Could you check a few things on this model? Use its own coordinates, in mm. A direction names the side the tool comes from. Round coordinates to 2 decimals unless told otherwise and drop trailing zeros. Loops run counter-clockwise (first coordinate to the right, second up) from the corner with the lowest first, then second, coordinate; pieces in that order, holes last. Notation, with made-up numbers: (-19.5, 71.5) -> (10.5, 71.5) arc R21 cw to (10.5, 96.5) -> close; hole circle Ø7 at (-38, 40). An arc over 180 degrees is marked (long way). Write each question's results on one line, items separated by ' | '. Start each with the question number.
1) Imagine slicing it at C-C, the plane x = -12. List the corners of the cut face in (y, z) for me, plus the area to 3 significant figures.
2) Imagine slicing it at B-B, the plane z = -4.25. List the corners of the cut face in (x, y) for me.
3) Which directions (+Z, -Z, +X, -X, +Y, -Y) give clear straight access to the entire face, cutting with the end or side of a thin tool? Please do faces 5 (the cylindrical face through (-10.24, -30.67, -4.93)), 6 (the flat face through (-9.857, -22, 4)), 7 (the flat face through (-24.857, -22, 1)).
4) If I drill on probe 1 along Z at (x, y) = (-19, -20); probe 2 along X at (y, z) = (-29.5, -3.75); probe 3 along Y at (x, z) = (-2.5, -5.25), over which ranges is the centre line in solid material (lowest first)?
5) Imagine slicing it at A-A, the plane y = -30. List the corners of the cut face in (x, z) for me.
6) We'd pull the mould along Y, two halves only. Please class faces 1 (the flat face through (-17, 0, 4)), 2 (the cylindrical face through (-17.59, -14.85, 4.03)), 3 (the flat face through (25.143, -22, -5)), 4 (the cylindrical face through (-3.585, -13.265, -4.93)): pulls with the +Y half, pulls with the -Y half, needs draft (parallel to the pull), parting line crosses it, or undercut.
7) Imagine slicing it at D-D, the plane y = -15. List the corners of the cut face in (x, z) for me, plus the area to 3 significant figures.
8) For P1, Ø5.5, axis at x = -3.36, y = -30, coming from the +Z side; P2, Ø0.6, axis at y = -25, z = 0.5, coming from the +X side; P3, Ø2, axis at y = -40, z = 3.5, coming from the +X side, each with a flat end and sliding along its axis, tell me the tip position at first contact or that it passes through.
from build123d import *

# Parameters (mm, degrees)
F0_W         = 15
F0_H         = 4
F1_DEPTH     = 44
F3_D         = 3.5
F4_R         = 1.75
F5_DEPTH     = 4
F7_D         = 4.2
F9_D         = 3.5
F9_DEPTH     = 10.001
F11_DEPTH    = 4
F12_T1_DEPTH = 69
F12_T3_DEPTH = 41


# Not quite as in the source:
# - a fillet or chamfer that OpenCascade refuses, or shapes differently, is made with other operations: its cross-section is extruded or revolved along the edge and cut away or added


with BuildPart() as f1:
    # F0 (on Front) → F1 (new body)
    with BuildSketch(Plane.XZ):
        Polygon((-28.8571389138, 6), (-28.8571389138, 0), (-24.8571389138, 0), (-24.8571389138, 2), (-24.8571389138, 6), align=None)
        Polygon((-24.8571389138, 0), (-28.8571389138, 0), (-28.8571389138, -10), (25.1428610862, -10), (25.1428610862, 0), align=None)
        with Locations((-17.3571389138, 4)):
            Rectangle(F0_W, F0_H)
    extrude(amount=F1_DEPTH)

    # F3 (through all)
    with Locations(Plane(origin=(0, 0, -10), x_dir=(1, 0, 0), z_dir=(0, 0, -1))):
        with Locations((-11.8571389138, 15), (-3.3571389138, 30)):
            Hole(F3_D / 2)

    # F4 (on face) → F5 (cut)
    with BuildSketch(Plane.XY.offset(6)):
        with BuildLine():
            Line((-9.8571389138, -20), (-9.8571389138, -10))
            ThreePointArc((-9.8571389138, -10), (-17.5900669637, -15), (-9.8571389138, -20))
        make_face()
        with Locations((-11.8571389138, -15)):
            Circle(F4_R, mode=Mode.SUBTRACT)
    extrude(amount=-F5_DEPTH, mode=Mode.SUBTRACT)

    # F7 (through all)
    with Locations(Plane.XZ.offset(44)):
        with Locations((-17.3571389138, -5)):
            Hole(F7_D / 2)

    # F9 (through all, one way)
    with BuildSketch(Plane.XY):
        with Locations((-3.3571389138, -15), (-11.8571389138, -30)):
            Circle(F9_D / 2)
    extrude(amount=-F9_DEPTH, mode=Mode.SUBTRACT)

    # F10 (on face) → F11 (cut, through all)
    with BuildSketch(Plane.XY.offset(6)):
        with BuildLine():
            Line((-9.8571389138, -35.1305356622), (-9.8571389138, -24.8694643378))
            ThreePointArc((-9.8571389138, -24.8694643378), (-17.3637164517, -30), (-9.8571389138, -35.1305356622))
        make_face()
    extrude(amount=-F11_DEPTH, mode=Mode.SUBTRACT)

    # F12: fillet of radius 5 on 4 edges, made by hand

    # F12_s2 → F12_t1 (cut)
    with BuildSketch(Plane.XZ.offset(-12.5)):
        with BuildLine():
            ThreePointArc((-28.8571389138, 1), (-27.3926728198, 4.5355339059), (-23.8571389138, 6))
            Line((-23.8571389138, 6), (-28.8571389138, 6))
            Line((-28.8571389138, 6), (-28.8571389138, 1))
        make_face()
        with BuildLine():
            ThreePointArc((-28.8571389138, -5), (-27.3926728198, -8.5355339059), (-23.8571389138, -10))
            Line((-23.8571389138, -10), (-28.8571389138, -10))
            Line((-28.8571389138, -10), (-28.8571389138, -5))
        make_face()
    extrude(amount=F12_T1_DEPTH, mode=Mode.SUBTRACT)

    # F12_s4 → F12_t3 (cut)
    with BuildSketch(Plane.XY.offset(-22.5)):
        with BuildLine():
            ThreePointArc((-28.8571389138, -5), (-27.3926728198, -1.4644660941), (-23.8571389138, 0))
            Line((-23.8571389138, 0), (-28.8571389138, 0))
            Line((-28.8571389138, 0), (-28.8571389138, -5))
        make_face()
        with BuildLine():
            ThreePointArc((-28.8571389138, -39), (-27.3926728198, -42.5355339059), (-23.8571389138, -44))
            Line((-23.8571389138, -44), (-28.8571389138, -44))
            Line((-28.8571389138, -44), (-28.8571389138, -39))
        make_face()
    extrude(amount=F12_T3_DEPTH, mode=Mode.SUBTRACT)


solid = f1.part
Checked values:
1) outline: (-44, -10) -> (-31.74, -10) -> (-31.74, 0) -> (-44, 0) -> close; (-44, 2) -> (-35.5, 2) -> (-35.5, 6) -> (-44, 6) -> close; (-28.26, -10) -> (-16.74, -10) -> (-16.74, 0) -> (-28.26, 0) -> close; (-24.5, 2) -> (-20.48, 2) -> (-20.48, 6) -> (-24.5, 6) -> close; (-13.26, -10) -> (0, -10) -> (0, 0) -> (-13.26, 0) -> close; (-9.52, 2) -> (0, 2) -> (0, 6) -> (-9.52, 6) -> close | area: 458 mm^2
2) outline: (-28.86, -39) arc R5 ccw to (-23.86, -44) -> (-19.32, -44) -> (-19.32, 0) -> (-23.86, 0) arc R5 ccw to (-28.86, -5) -> close; (-15.4, -44) -> (25.14, -44) -> (25.14, 0) -> (-15.4, 0) -> close; hole circle Ø3.5 at (-11.86, -30); hole circle Ø3.5 at (-11.86, -15); hole circle Ø3.5 at (-3.36, -30); hole circle Ø3.5 at (-3.36, -15)
3) face 5: +Z, -Z | face 6: +Z, +X, +Y, -Y | face 7: +X, +Y, -Y
4) probe 1: -10 to -6.31, -3.69 to 0, 2 to 6 | probe 2: -28.86 to -19.04, -15.67 to -13.53, -10.18 to -5.03, -1.68 to 25.14 | probe 3: -44 to -31.53, -28.47 to -16.53, -13.47 to 0
5) outline: (-28.86, -5) arc R5 ccw to (-23.86, -10) -> (-13.61, -10) -> (-13.61, 0) -> (-24.86, 0) -> (-24.86, 2) -> (-17.36, 2) -> (-17.36, 6) -> (-23.86, 6) arc R5 ccw to (-28.86, 1) -> close; (-10.11, -10) -> (-5.11, -10) -> (-5.11, 0) -> (-10.11, 0) -> close; (-1.61, -10) -> (25.14, -10) -> (25.14, 0) -> (-1.61, 0) -> close; hole circle Ø4.2 at (-17.36, -5)
6) face 1: pulls with the +Y half | face 2: undercut | face 3: needs draft | face 4: undercut
7) outline: (-28.86, -5) arc R5 ccw to (-23.86, -10) -> (-13.61, -10) -> (-13.61, 0) -> (-24.86, 0) -> (-24.86, 2) -> (-17.59, 2) -> (-17.59, 6) -> (-23.86, 6) arc R5 ccw to (-28.86, 1) -> close; (-10.11, -10) -> (-5.11, -10) -> (-5.11, 0) -> (-10.11, 0) -> close; (-1.61, -10) -> (25.14, -10) -> (25.14, 0) -> (-1.61, 0) -> close; hole circle Ø4.2 at (-17.36, -5) | area: 498 mm^2
8) P1: z = 0 | P2: x = -24.86 | P3: x = -9.86
